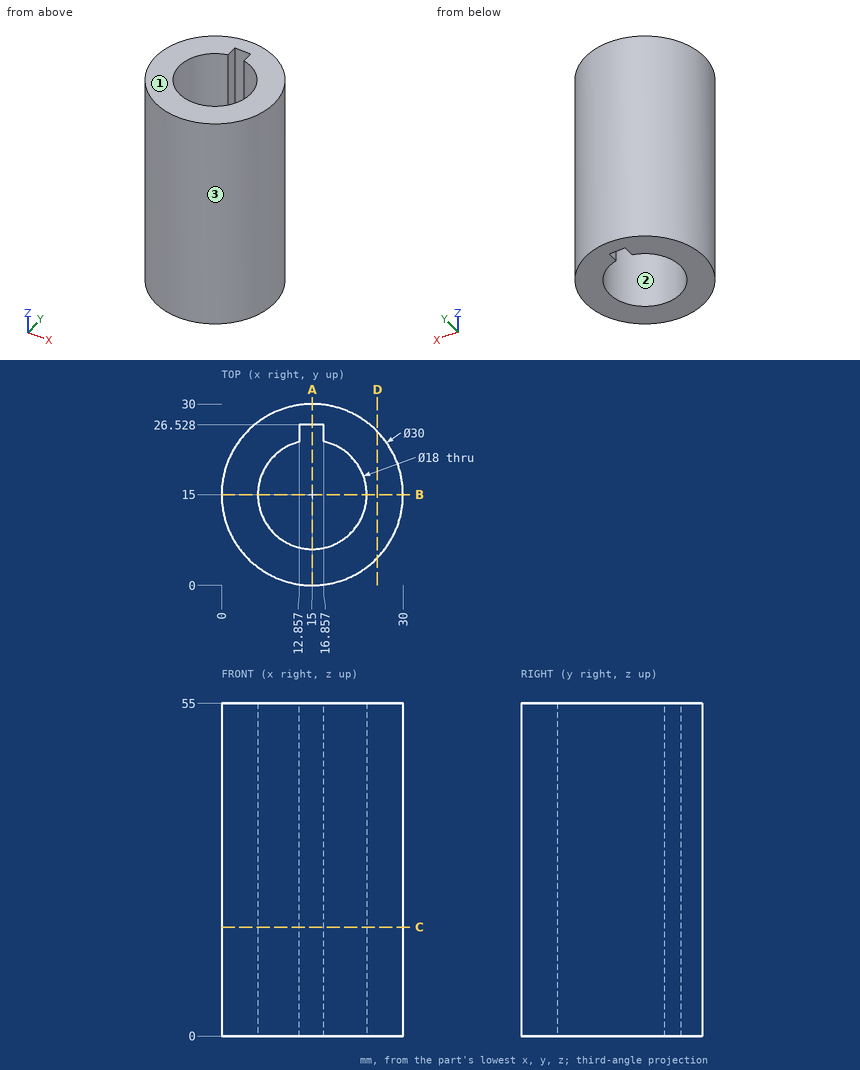
Input: dimensioned drawing with shaded views. Units: mm. Origin: part minimum x, y, z. Coordinates: 2 decimals unless noted, no trailing zeros. Loops run counter-clockwise (first coordinate to the right, second up) from the corner with the lowest first, then second, coordinate; pieces in that order, holes last. Notation, with made-up numbers: (67, 61.25) - (110, 61.25) arc R29 cw to (110, 83.25) - close; hole circle Ø10 at (85, 11.25). An arc over 180 degrees is marked (long way). One line per question, with ' | ' between items. Start each with the question number.
(1) Draft query along X for the marked faces 1, 2 and 3. Return one class per face: +X half, -X half, draft (parallel to the pull), parting line (faces both ways), or undercut.
(2) Ray query, L1, parallel to Y at x = 15, z = 25; L2, parallel to X at y = 15.25, z = 20.5; L3, parallel to X at y = 13.25, z = 29.5. Return the intervals inside material, ascending. Write a range as from..to.
(3) Cut plane D-D on x = 25.75. Output: boundary loops of the cut face in (y, z), and give its area (3 significant figures).
(4) Cut plane B-B on y = 15. Output: boundary loops of the cut face in (x, z), and give its area (3 significant figures).
(5) First-contact query: pin 1 (3 mm diameter, centred on y = 9, z = 23, fed in from +X); pin 2 (1 mm diameter, centred on x = 4, y = 5, fed in from -Z); pin 3 (1 mm diameter, centred on y = 10, z = 12, fed in from -X); pin 4 (4 mm diameter, centred on y = 6.5, z = 37.5, fed in from -X). Flat tips, straight axial feed; report the tip coordinate or a pass-through.
(6) Cut plane C-C on z = 18. Output: boundary loops of the cut face in (x, y), and give its area (3 significant figures).
(7) Cut plane A-A on x = 15. Output: boundary loops of the cut face in (y, z), and give its area (3 significant figures).
Here are the results:
1) face 1: draft | face 2: undercut | face 3: parting line
2) L1: 0..6, 26.53..30 | L2: 0..6, 24..30 | L3: 0.1..6.17, 23.83..29.9
3) outline: (4.54, 0) - (25.46, 0) - (25.46, 55) - (4.54, 55) - close | area: 1,150 mm²
4) outline: (0, 0) - (6, 0) - (6, 55) - (0, 55) - close; (24, 0) - (30, 0) - (30, 55) - (24, 55) - close | area: 660 mm²
5) pin 1: x = 29.31 | pin 2: z = 0 | pin 3: x = 0.69 | pin 4: x = 1.48
6) outline: circle Ø30 at (15, 15); hole (12.86, 23.74) arc R9 ccw (long way) to (16.86, 23.81) - (16.86, 26.53) - (12.86, 26.53) - close | area: 442 mm²
7) outline: (0, 0) - (6, 0) - (6, 55) - (0, 55) - close; (26.53, 0) - (30, 0) - (30, 55) - (26.53, 55) - close | area: 521 mm²
